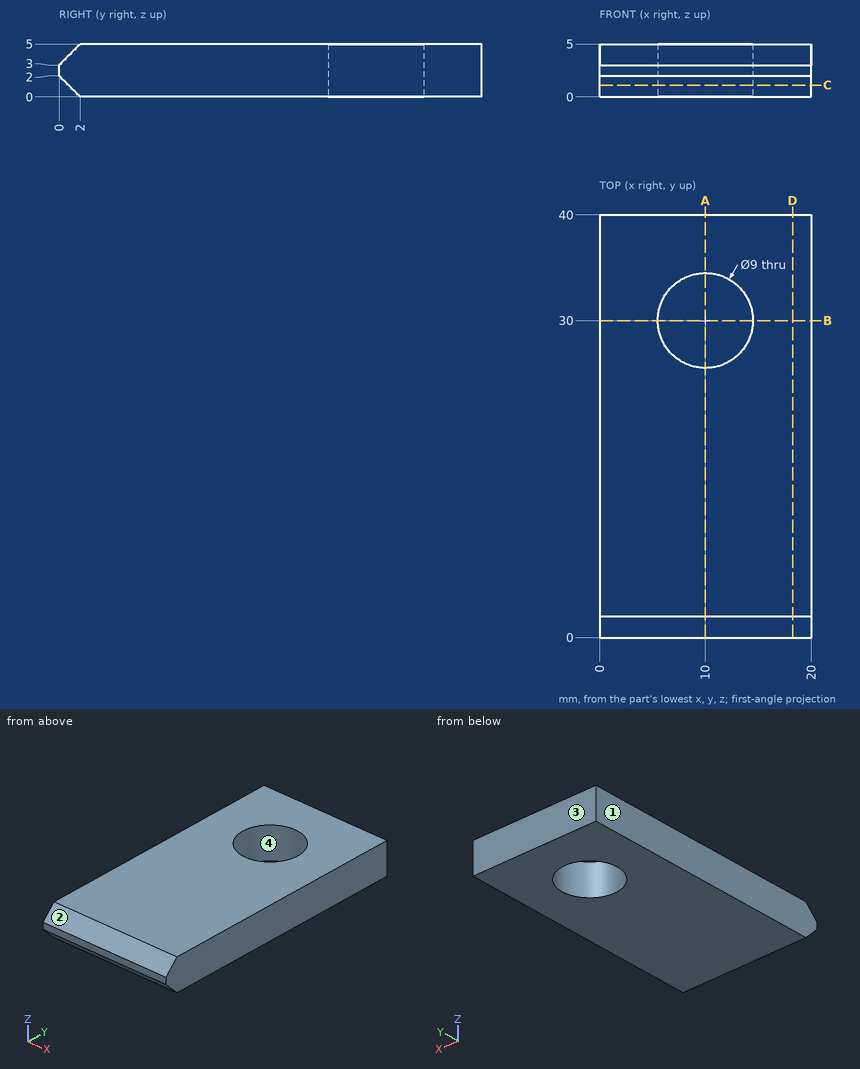
Geometry check sheet. Reference: drawing and pictorial views, mm from the part's lowest x, y, z. Give positions to 0.01 mm unless a question says otherwise; leave off trailing zeros. Loops run counter-clockwise (first coordinate to the right, second up) from the corner with the lowest first, then second, coordinate; pieces in that order, holes last. Notation, with made-up numbers: M -13,-33.75 L -8,-33.75 A17 cw -8,-17.75 Z; hole C 19,30 d7. An arc over 180 degrees is marked long. Use a Markdown table: item, result. Add a question column.
Q1. Mould release check, pull along Y, two halves, no side actions. Record for the marked faces 1, 2, 3 and 4: pulls with the +Y half, pulls with the -Y half, needs draft (parallel to the pull), parting line crosses it, or undercut.
Q2. Sectioned sample at A-A, the plane x = 10. Record the cut outline in (y, z), then the cut area to 3 significant figures.
Q3. Sectioned sample at C-C, the plane z = 1.1. Record the cut outline in (x, y), then the cut area to 3 significant figures.
Q4. Sectioned sample at B-B, the plane y = 30. Record the cut outline in (x, z).
Q5. Scan lines: line 1 along Y through (x, z) = (14, 0.55); line 2 along Y through (x, z) = (10, 3.6); line 3 along X through (y, z) = (28.5, 3). Record each from-to range of solid material in increasing order. Write a range as [from, to].
Q6. Sectioned sample at D-D, the plane x = 18.25. Record the cut outline in (y, z), then the cut area to 3 significant figures.
Verdict:
| question | item | result |
|---|---|---|
| 1 | face 1 | needs draft |
| 1 | face 2 | pulls with the -Y half |
| 1 | face 3 | pulls with the +Y half |
| 1 | face 4 | undercut |
| 2 | outline | M 0,2 L 2,0 L 25.5,0 L 25.5,5 L 2,5 L 0,3 Z; M 34.5,0 L 40,0 L 40,5 L 34.5,5 Z |
| 2 | area | 151 mm^2 |
| 3 | outline | M 0,0.9 L 20,0.9 L 20,40 L 0,40 Z; hole C 10,30 d9 |
| 3 | area | 718 mm^2 |
| 4 | outline | M 0,0 L 5.5,0 L 5.5,5 L 0,5 Z; M 14.5,0 L 20,0 L 20,5 L 14.5,5 Z |
| 5 | line 1 | [1.45, 27.94], [32.06, 40] |
| 5 | line 2 | [0.6, 25.5], [34.5, 40] |
| 5 | line 3 | [0, 5.76], [14.24, 20] |
| 6 | outline | M 0,2 L 2,0 L 40,0 L 40,5 L 2,5 L 0,3 Z |
| 6 | area | 196 mm^2 |
